Here's how the part is built. I have some questions about the finished solid (model axes, mm). Face numbers are marked on the shaded views. Coordinates: 2 decimals unless noted, no trailing zeros. Write each loop counter-clockwise with the first axis right and the second up, starting at its lowest first coordinate (ties: lowest second). Pieces come first, ordered by that corner, then holes.
Item 1: If we section it at D-D (z = -40): Please give me the cut outline in (x, y), then the cut area to 3 significant figures.
Item 2: We'd pull the mould along Z, two halves only. Please class the marked faces 1, 2 and 3: +Z half, -Z half, draft (parallel to the pull), parting line (faces both ways), or undercut.
Item 3: If we section it at C-C (x = 5.5): Please give me the cut outline in (y, z).
Item 4: If I drill on line 1 (Z direction, x = 9, y = 1.5); line 2 (X direction, y = 4.5, z = -38); line 3 (X direction, y = 5, z = 19), over which ranges is the centre line in solid material (lowest first)?
Item 5: If we section it at A-A (z = -59.5): Please give me the cut outline in (x, y), then the cut area to 3 significant figures.
Item 6: If we section it at B-B (y = 5): Please give me the cut outline in (x, z).
Item 7: I'm going to push flat-ended pins straight in: pin 1 Ø2.5 at (x, z) = (1, -1) entering from -Y; pin 2 Ø3 at (y, z) = (4, 18.5) entering from -X; pin 3 Ø2.5 at (y, z) = (-15, 39) entering from +X; pin 4 Ø11 at (x, y) = (18.5, 5.5) entering from +Z. Where does each tip first touch, or does it pass through?
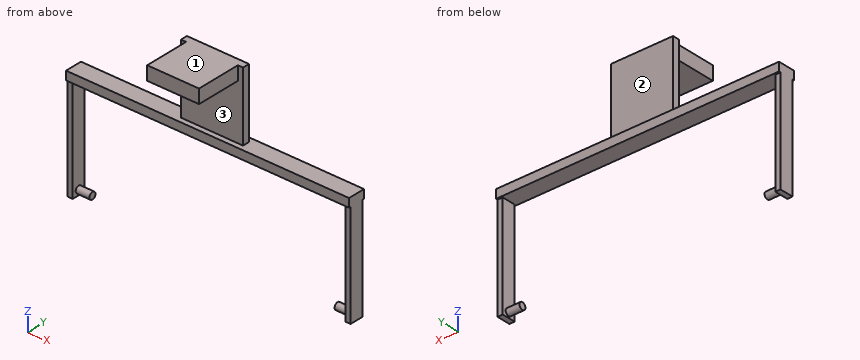
from build123d import *

# Parameters (mm, degrees)
SKETCH_1_W             = 164
SKETCH_1_H             = 5
EXTRUDE_1_DEPTH        = 10
SKETCH_2_W             = 3
SKETCH_2_H             = 8
EXTRUDE_2_DEPTH        = 60
PATTERN_LINEAR_1_COUNT = 2
PATTERN_LINEAR_1_PITCH = 161
SKETCH_4_R             = 2
EXTRUDE_3_DEPTH        = 8
EXTRUDE_START          = 8
SKETCH_5_R             = 2
EXTRUDE_4_DEPTH        = 8
SKETCH_6_W             = 36
SKETCH_6_H             = 4
EXTRUDE_5_DEPTH        = 40
SKETCH_7_W             = 30
SKETCH_7_H             = 8
EXTRUDE_6_DEPTH        = 26


with BuildPart() as part:
    # 草图1 → 凸台-拉伸1 (new body)
    with BuildSketch(Plane(origin=(0, 0, 0), x_dir=(1, 0, 0), z_dir=(0, 1, 0))):
        Rectangle(SKETCH_1_W, SKETCH_1_H)
    extrude(amount=EXTRUDE_1_DEPTH)

    # 草图2 → 凸台-拉伸2 (add)
    with BuildSketch(Plane(origin=(0, 0, -2.5), x_dir=(-1, 0, 0), z_dir=(0, 0, -1))):
        with Locations((-80.5, 5)):
            Rectangle(SKETCH_2_W, SKETCH_2_H)
    extrude_2 = extrude(amount=EXTRUDE_2_DEPTH)

    # 阵列(线性)1: 凸台-拉伸2 ×2
    with Locations(*[(-i * PATTERN_LINEAR_1_PITCH, 0, 0) for i in range(1, PATTERN_LINEAR_1_COUNT)]):
        add(extrude_2)

    # 草图4 → 凸台-拉伸3 (add)
    with BuildSketch(Plane(origin=(-79, 0, 0), x_dir=(0, 0, -1), z_dir=(1, 0, 0))):
        with Locations(Location((59.5, 5, 0), (0, 0, 180))):
            Circle(SKETCH_4_R)
    extrude(amount=EXTRUDE_3_DEPTH)

    # 草图5 → 凸台-拉伸4 (add)
    with BuildSketch(Plane.ZY.offset(-79).offset(EXTRUDE_START)):
        with Locations((-59.5, 5)):
            Circle(SKETCH_5_R)
    extrude(amount=-EXTRUDE_4_DEPTH)

    # 草图6 → 凸台-拉伸5 (add)
    with BuildSketch(Plane.XY.offset(2.5)):
        with Locations((0, 5)):
            Rectangle(SKETCH_6_W, SKETCH_6_H)
    extrude(amount=EXTRUDE_5_DEPTH)

    # 草图7 → 凸台-拉伸6 (add)
    with BuildSketch(Plane.XZ.offset(-3)):
        with Locations((0, 38.5)):
            Rectangle(SKETCH_7_W, SKETCH_7_H)
    extrude(amount=EXTRUDE_6_DEPTH)


solid = part.part
Answer list:
1. outline: (-82, 1) - (-79, 1) - (-79, 9) - (-82, 9) - close; (79, 1) - (82, 1) - (82, 9) - (79, 9) - close
1. area: 48.0 mm2
2. face 1: +Z half
2. face 2: draft
2. face 3: undercut
3. outline: (-23, 34.5) - (3, 34.5) - (3, 2.5) - (0, 2.5) - (0, -2.5) - (10, -2.5) - (10, 2.5) - (7, 2.5) - (7, 42.5) - (-23, 42.5) - close
4. line 1: z = -2.5 to 2.5, 34.5 to 42.5
4. line 2: x = -82 to -79, 79 to 82
4. line 3: x = -18 to 18
5. outline: (-82, 1) - (-79, 1) - (-79, 3) - (-71, 3) - (-71, 7) - (-79, 7) - (-79, 9) - (-82, 9) - close; (71, 3) - (79, 3) - (79, 1) - (82, 1) - (82, 9) - (79, 9) - (79, 7) - (71, 7) - close
5. area: 112 mm2
6. outline: (-82, -62.5) - (-79, -62.5) - (-79, -61.5) - (-71, -61.5) - (-71, -57.5) - (-79, -57.5) - (-79, -2.5) - (79, -2.5) - (79, -57.5) - (71, -57.5) - (71, -61.5) - (79, -61.5) - (79, -62.5) - (82, -62.5) - (82, 2.5) - (18, 2.5) - (18, 42.5) - (-18, 42.5) - (-18, 2.5) - (-82, 2.5) - close
7. pin 1: stops at y = 0
7. pin 2: stops at x = -18
7. pin 3: stops at x = 15
7. pin 4: stops at z = 42.5
